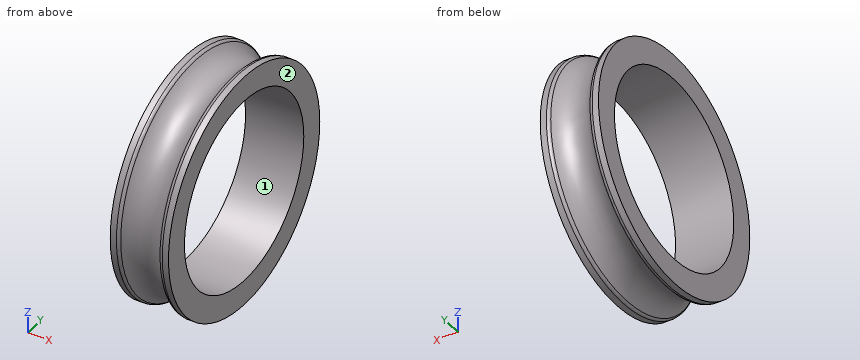
from build123d import *

# Parameters (mm, degrees)
F2_R = 0.5


with BuildPart() as f1:
    # F0 (on Top) → F1 (revolve)
    with BuildSketch(Plane.XY):
        with BuildLine():
            Line((-3.5, -1.5), (3.5, -1.5))
            Line((3.5, -1.5), (3.5, 1.5))
            Line((3.5, 1.5), (2.5, 1.5))
            ThreePointArc((2.5, 1.5), (0, 0.1583123952), (-2.5, 1.5))
            Line((-2.5, 1.5), (-3.5, 1.5))
            Line((-3.5, 1.5), (-3.5, -1.5))
        make_face()
    revolve(axis=Axis((0, -12.7, 0), (1, 0, 0)))

    # F2
    f2_edges = [f1.edges().sort_by_distance(p)[0] for p in [
        (-2.5, -26.9, 0),
        (2.5, -26.9, 0),
    ]]
    fillet(f2_edges, radius=F2_R)


solid = f1.part
Read the model definition and answer for the solid it produces. Units are mm, in the model's axes. Face numbers are marked on the shaded views. Coordinates: 2 decimals unless noted, no trailing zeros. Write each loop counter-clockwise with the first axis right and the second up, starting at its lowest first coordinate (ties: lowest second). Pieces come first, ordered by that corner, then holes. Notation, with made-up numbers: (46, -11.75) -> (84, -11.75) arc R16 ccw to (84, 8.25) -> close; hole circle Ø3 at (84, -12.5). An arc over 180 degrees is marked (long way). Return JSON: item names as keys, results as strings.
(1) Consider line 1 along Z through (x, y) = (1.5, -12.7); line 2 along Z through (x, y) = (-1, -12.7); line 3 along Y through (x, z) = (1.5, 0.25). Determine where each line is inside the solid, lowest interval first. Write a range as from..to.
Answers below:
{"line 1": "-13.26..-11.2, 11.2..13.26", "line 2": "-13.03..-11.2, 11.2..13.03", "line 3": "-25.96..-23.9, -1.5..0.56"}
(2) The part is cut by section A-A on x = 1. Give the vertices of the cut face in (y, z).
Answers below:
{"outline": "circle Ø26.06 at (-12.7, 0); hole circle Ø22.4 at (-12.7, 0)"}
(3) For a pull along Y with two mould halves and no side action, classify the marked faces 1 and 2 as pulls with the +Y half, pulls with the -Y half, needs draft (parallel to the pull), parting line crosses it, or undercut.
Answers below:
{"face 1": "undercut", "face 2": "needs draft"}
(4) Each of these flat-tipped pins is pushed along its axis until it touches: P1, Ø10, axis at y = -3, z = 0, coming from the +X side; P2, Ø1, axis at x = -1, z = 9, coming from the -Y side; P3, Ø1.5, axis at x = 1, z = 4.5, coming from the +Y side. Where does it stop, or does it pass through?
Answers below:
{"P1": "x = 3.5", "P2": "y = -22.65", "P3": "y = 0"}
